```python
from build123d import *

# Parameters (mm, degrees)
F0_W      = 50.4
F0_H      = 38.8
F1_DEPTH  = 1.6
F2_W      = 18.75
F2_H      = 15
F3_DEPTH  = 15.5
F4_W      = 7.75
F4_H      = 30
F5_DEPTH  = 10
F6_SIZE2  = 3.5
F6_SIZE   = 3.5
F7_W      = 2.5
F7_H      = 9.85
F8_DEPTH  = 17
F9_R      = 2.5
F10_R     = 1.6
F11_DEPTH = 1.601


with BuildPart() as f1:
    # F0 (on Top) → F1 (new body)
    with BuildSketch(Plane.XY):
        Rectangle(F0_W, F0_H)
    extrude(amount=F1_DEPTH)

    # F2 (on face) → F3 (join)
    with BuildSketch(Plane.XY.offset(1.6)):
        with Locations((3.575, -9.9)):
            Rectangle(F2_W, F2_H)
        with Locations((3.575, 7.1)):
            Rectangle(F2_W, F2_H)
    extrude(amount=F3_DEPTH)

    # F4 (on face) → F5 (join)
    with BuildSketch(Plane.XY.offset(1.6)):
        with Locations((17.625, -1.4)):
            Rectangle(F4_W, F4_H)
    extrude(amount=F5_DEPTH)

    # F6
    f6_edges = [f1.edges().sort_by_distance(p)[0] for p in [
        (13.75, -1.4, 11.6),
    ]]
    chamfer(f6_edges, length=F6_SIZE, length2=F6_SIZE2)

    # F7 (on face) → F8 (join)
    with BuildSketch(Plane.XY.offset(1.6)):
        with Locations((-22.7, -7.675)):
            Rectangle(F7_W, F7_H)
    extrude(amount=F8_DEPTH)

    # F9
    f9_edges = [f1.edges().sort_by_distance(p)[0] for p in [
        (-25.2, 19.4, 0.8),
        (25.2, 19.4, 0.8),
        (25.2, -19.4, 0.8),
        (-25.2, -19.4, 0.8),
    ]]
    fillet(f9_edges, radius=F9_R)

    # F10 (on face) → F11 (cut, through all)
    with BuildSketch(Plane.XY.offset(1.6)):
        with Locations((-22.7, 16.9)):
            Circle(F10_R)
        with Locations((22.7, 16.9)):
            Circle(F10_R)
        with Locations((22.7, -16.9)):
            Circle(F10_R)
        with Locations((-22.7, -16.9)):
            Circle(F10_R)
    extrude(amount=-F11_DEPTH, mode=Mode.SUBTRACT)


solid = f1.part
```
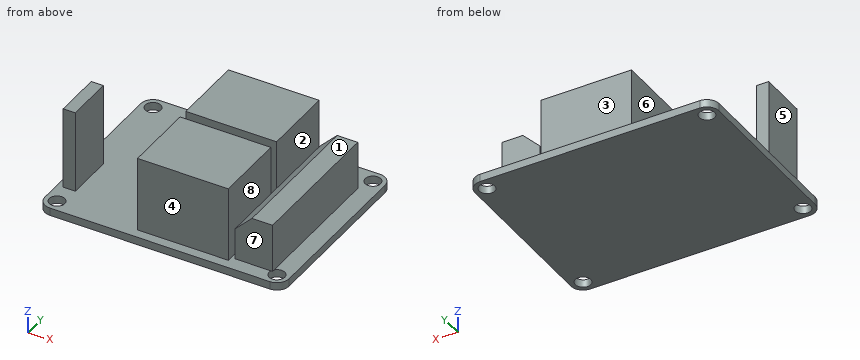
Build history of the part. All positions in model axes, mm. Face numbers are marked on the shaded views. A direction names the side the tool comes from. Coordinates: 2 decimals unless noted, no trailing zeros. Order: outer loops, then holes, each group sorted by start corner. A loop starts at its lowest first (then second) coordinate and runs counter-clockwise, first axis right, second up.
Item 1: Saw through at A-A on z = 9.25. List the corners of the cut face in (x, y).
Filled in:
outline: (-23.95, -12.6) - (-21.45, -12.6) - (-21.45, -2.75) - (-23.95, -2.75) - close; (-5.8, -17.4) - (12.95, -17.4) - (12.95, -2.4) - (-5.8, -2.4) - close; (-5.8, -0.4) - (12.95, -0.4) - (12.95, 14.6) - (-5.8, 14.6) - close; (14.9, -16.4) - (21.5, -16.4) - (21.5, 13.6) - (14.9, 13.6) - close
Item 2: Drill centre lines: L1, parallel to Y at x = -22.7, z = 0.8; L2, parallel to Y at x = 11.5, z = 8; L3, parallel to X at y = 11, z = 2.5. Where is each one in solid material? Low to high.
Filled in:
L1: y = -19.4 to -18.5, -15.3 to 15.3, 18.5 to 19.4
L2: y = -17.4 to -2.4, -0.4 to 14.6
L3: x = -5.8 to 12.95, 13.75 to 21.5
Item 3: Tool access for the marked faces 1, 2, 3, 4 and 5: list every direction of +Z, -Z, +X, -X, +Y, -Y with a clear straight run to the whole face (end or side of a thin tool).
Filled in:
face 1: +Z, +X, +Y, -Y
face 2: +Z, +Y, -Y
face 3: +Z, +X, -X, +Y
face 4: +Z, +X, -X, -Y
face 5: +Z, -X, +Y, -Y
Item 4: Mould opens along X. For the marked faces 6, 7 and 8 say: released by +X, released by -X, zero draft, split by the parting line, or undercut.
Filled in:
face 6: released by -X
face 7: zero draft
face 8: undercut
Item 5: Saw through at D-D on x = 19. List the corners of the cut face in (y, z).
Filled in:
outline: (-19.4, 0) - (19.4, 0) - (19.4, 1.6) - (13.6, 1.6) - (13.6, 11.6) - (-16.4, 11.6) - (-16.4, 1.6) - (-19.4, 1.6) - close
Item 6: Drop flat-ended pins along their axis: pin 1 Ø4.5 at (y, z) = (-12.5, 10.5) entering from -X; pin 2 Ø8 at (y, z) = (-6, 10.5) entering from +X; pin 3 Ø1.5 at (x, y) = (-10.5, 4.5) entering from +Z. Give the stop position or say it passes through.
Filled in:
pin 1: stops at x = -23.95
pin 2: stops at x = 21.5
pin 3: stops at z = 1.6
Item 7: Saw through at B-B on z = 14.5. List the corners of the cut face in (x, y).
Filled in:
outline: (-23.95, -12.6) - (-21.45, -12.6) - (-21.45, -2.75) - (-23.95, -2.75) - close; (-5.8, -17.4) - (12.95, -17.4) - (12.95, -2.4) - (-5.8, -2.4) - close; (-5.8, -0.4) - (12.95, -0.4) - (12.95, 14.6) - (-5.8, 14.6) - close
Item 8: Saw through at C-C on y = 5. List the corners of the cut face in (x, z), then the cut area to 3 significant figures.
Filled in:
outline: (-25.2, 0) - (25.2, 0) - (25.2, 1.6) - (21.5, 1.6) - (21.5, 11.6) - (17.25, 11.6) - (13.75, 8.1) - (13.75, 1.6) - (12.95, 1.6) - (12.95, 17.1) - (-5.8, 17.1) - (-5.8, 1.6) - (-25.2, 1.6) - close
area: 443 mm2
